Part model, mm, in its own coordinate system. A direction names the side the tool comes from. Coordinates: 2 decimals unless noted, no trailing zeros. Loops run counter-clockwise (first coordinate to the right, second up) from the corner with the lowest first, then second, coordinate; pieces in that order, holes last. Notation, with made-up numbers: M -17.75,9 L -11.75,9 A19 cw -11.75,39 Z; hole C 87,-20 d8. An arc over 180 degrees is marked long. Answer as CSV lines item,"result". Start each with the question number.
from build123d import *

# Parameters (mm, degrees)
SKETCH1_W            = 120
SKETCH1_H            = 140
SKETCH1_R            = 52.5
BOSS_EXTRUDE1_DEPTH  = 4
M4_CLEARANCE_HOLE1_D = 4.5
M5_CLEARANCE_HOLE1_D = 5.5
BOSS_EXTRUDE2_DEPTH  = 4
FILLET1_R            = 3


with BuildPart() as part:
    # Sketch1 → Boss-Extrude1 (new body)
    with BuildSketch(Plane.XY):
        with Locations((60, 70)):
            Rectangle(SKETCH1_W, SKETCH1_H)
        with Locations((60, 60)):
            Circle(SKETCH1_R, mode=Mode.SUBTRACT)
    extrude(amount=BOSS_EXTRUDE1_DEPTH)

    # M4 Clearance Hole1 (through all)
    with Locations(Plane.XY.offset(4)):
        with Locations((7.5, 7.5), (60, 60), (7.5, 112.5), (112.5, 112.5), (112.5, 7.5)):
            Hole(M4_CLEARANCE_HOLE1_D / 2)

    # M5 Clearance Hole1 (through all)
    with Locations(Plane.XY.offset(4)):
        with Locations((100, 130), (20, 130)):
            Hole(M5_CLEARANCE_HOLE1_D / 2)

    # Sketch6 → Boss-Extrude2 (add)
    with BuildSketch(Plane(origin=(120, 0, 0), x_dir=(0, 0, -1), z_dir=(1, 0, 0))):
        Polygon((-4, 140), (7.829119834, 140), (11, 136.829119834), (11, 105), (0, 0), (-4, 0), align=None)
    boss_extrude2 = extrude(amount=BOSS_EXTRUDE2_DEPTH)

    # Mirror1: Boss-Extrude2 across plane
    add(boss_extrude2.mirror(Plane.ZY.offset(-60)))

    # Fillet1
    fillet1_edges = [part.edges().sort_by_distance(p)[0] for p in [
        (120, 70, 0),
        (0, 70, 0),
    ]]
    fillet(fillet1_edges, radius=FILLET1_R)


solid = part.part
Q1. Flat gauge pin, fed straight in: P1, Ø7, axis at x = 7.5, y = 7.5, coming from the -Z side. Where does the tip first touch, or does it go through?
Q2. Wall check: L1, parallel to X at y = 78, z = -4.5; L2, parallel to Y at x = 100, z = 2.65; L3, parallel to X at y = 114.5, z = 1.5. Give the ranges that are in metal, low to high.
Q3. Slice it at A-A, the plane x = 60. Write the cut outline in (y, z), and give its area (3 significant figures).
Q4. Slice it at D-D, the plane x = 100. Write the cut outline in (y, z).
Q5. Tool access for faces 4 (the face through (100.596, 127.315, 1.972)), 5 (the face through (120, 97, -6)): list every direction of +Z, -Z, +X, -X, +Y, -Y with a clear straight run to the whole face (end or side of a thin tool).
Q6. Slice it at B-B, the plane y = 64. Write the cut outline in (x, z).
Q7. Two-plate mould, pull along Y, no slides. Class faces 1 (the face through (60, 140, 2)), 2 (the face through (-4, 87, -2)), 3 (the face through (7.988, 110.304, 1.972)): +Y half, -Y half, draft (parallel to the pull), parting line (faces both ways), or undercut.
Q8. Slice it at C-C, the plane y = 130. Write the cut outline in (x, z), and give its area (3 significant figures).
Solved:
1,P1,"stops at z = 0"
2,L1,"x = -4 to 0, 120 to 124"
2,L2,"y = 0 to 26, 94 to 127.25, 132.75 to 140"
2,L3,"x = -4 to 6.47, 8.53 to 111.47, 113.53 to 124"
3,outline,"M 0,0 L 7.5,0 L 7.5,4 L 0,4 Z; M 112.5,0 L 140,0 L 140,4 L 112.5,4 Z"
3,area,"140 mm2"
4,outline,"M 0,0 L 26,0 L 26,4 L 0,4 Z; M 94,0 L 127.25,0 L 127.25,4 L 94,4 Z; M 132.75,0 L 140,0 L 140,4 L 132.75,4 Z"
5,face 4,"+Z, -Z"
5,face 5,"-Z, +Y, -Y"
6,outline,"M -4,-6.7 L 0,-6.7 L 0,-3 A3 cw 3,0 L 7.65,0 L 7.65,4 L -4,4 Z; M 112.35,0 L 117,0 A3 cw 120,-3 L 120,-6.7 L 124,-6.7 L 124,4 L 112.35,4 Z"
7,face 1,"+Y half"
7,face 2,"draft"
7,face 3,"undercut"
8,outline,"M -4,-11 L 0,-11 L 0,-3 A3 cw 3,0 L 17.25,0 L 17.25,4 L -4,4 Z; M 22.75,0 L 97.25,0 L 97.25,4 L 22.75,4 Z; M 102.75,0 L 117,0 A3 cw 120,-3 L 120,-11 L 124,-11 L 124,4 L 102.75,4 Z"
8,area,"560 mm2"
